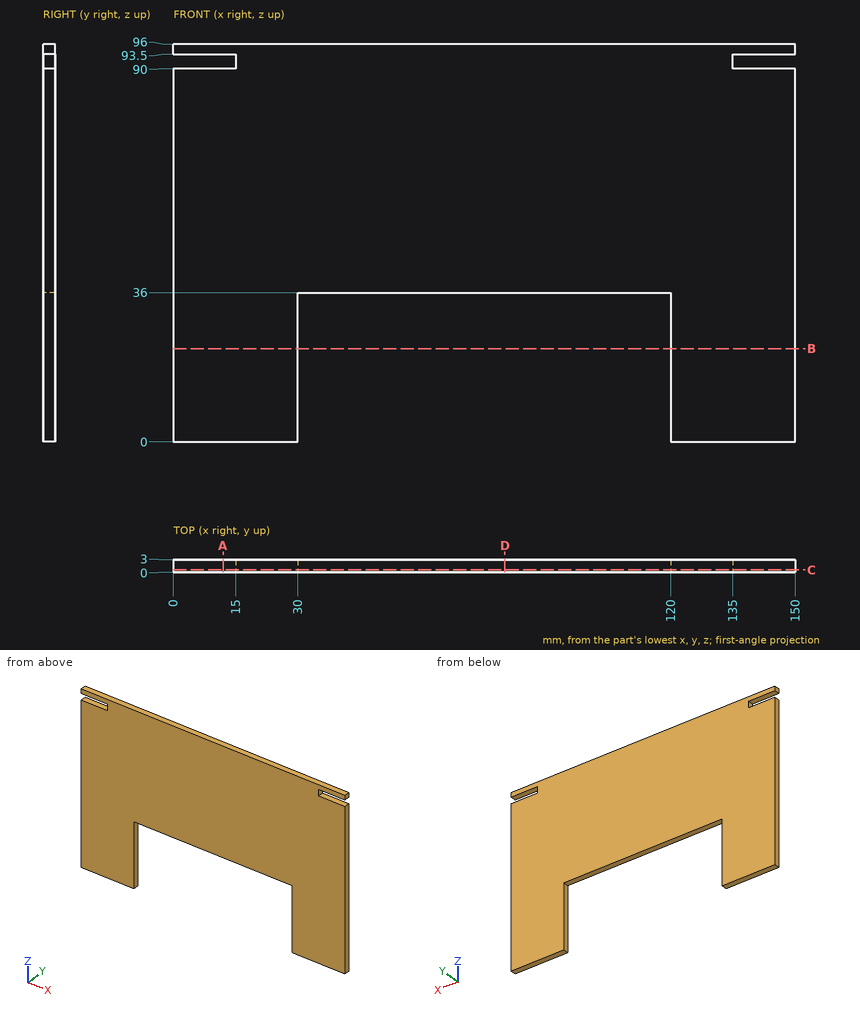
Geometry check sheet. Reference: drawing and pictorial views, mm from the part's lowest x, y, z. Give positions to 0.01 mm unless a question says otherwise; leave off trailing zeros. Order: outer loops, then holes, each group sorted by start corner. A loop starts at its lowest first (then second) coordinate and runs counter-clockwise, first axis right, second up. Notation, with made-up numbers: (52.5, -30) -> (96.5, -30) arc R21 ccw to (96.5, 1) -> close; hole circle Ø2 at (-25.75, 19). An arc over 180 degrees is marked (long way). Write each question's results on one line, items separated by ' | '. Start each with the question number.
(1) Scan lines: line 1 (X direction, y = 1.7, z = 13.5); line 2 (Z direction, x = 48.5, y = 1.25); line 3 (Z direction, x = 13.5, y = 0.25). Record each from-to range of solid material in increasing order.
(2) Sectioned sample at A-A (x = 12). Enter the section's corners in (y, z), plus the area to 4 significant figures.
(3) Sectioned sample at B-B (z = 22.5). Enter the section's corners in (x, y), plus the area to 3 significant figures.
(4) Sectioned sample at D-D (x = 80). Enter the section's corners in (y, z).
(5) Sectioned sample at C-C (y = 0.55). Enter the section's corners in (x, z), plus the area to 3 significant figures.
(6) Gauge pin test, flat ends, axial feed: P1, Ø0.9, axis at y = 1.5, z = 91, coming from the +X side; P2, Ø0.9, axis at y = 1, z = 92.5, coming from the -X side; P3, Ø1.5, axis at x = 90, y = 1.5, coming from the -Z side. Record the tip position at first contact, or that the pin passes through.
Answer below:
1) line 1: 0 to 30, 120 to 150 | line 2: 36 to 96 | line 3: 0 to 90, 93.5 to 96
2) outline: (0, 0) -> (3, 0) -> (3, 90) -> (0, 90) -> close; (0, 93.5) -> (3, 93.5) -> (3, 96) -> (0, 96) -> close | area: 277.5 mm2
3) outline: (0, 0) -> (30, 0) -> (30, 3) -> (0, 3) -> close; (120, 0) -> (150, 0) -> (150, 3) -> (120, 3) -> close | area: 180 mm2
4) outline: (0, 36) -> (3, 36) -> (3, 96) -> (0, 96) -> close
5) outline: (0, 0) -> (30, 0) -> (30, 36) -> (120, 36) -> (120, 0) -> (150, 0) -> (150, 90) -> (135, 90) -> (135, 93.5) -> (150, 93.5) -> (150, 96) -> (0, 96) -> (0, 93.5) -> (15, 93.5) -> (15, 90) -> (0, 90) -> close | area: 11,100 mm2
6) P1: x = 135 | P2: x = 15 | P3: z = 36
